Source: CAD feature listing. Evaluate the final solid. Frame: model axes, mm. Give positions to 0.01 mm unless a question says otherwise; leave off trailing zeros. Order: outer loops, then holes, each group sorted by start corner. A loop starts at its lowest first (then second) coordinate and runs counter-clockwise, first axis right, second up.
1) Section C-C, the plane y = 5. Return loops of the section in (x, z).
2) First-contact query: P1, Ø1, axis at x = 1.5, y = -6, coming from the -Z side; P2, Ø1, axis at x = 3, z = 2.5, coming from the -Y side. Flat tips, straight axial feed; report the tip coordinate or a pass-through.
3) Section D-D, the plane z = 2.75. Return loops of the section in (x, y).
4) Section A-A, the plane z = 1.3. Return loops of the section in (x, y), plus the area to 3 significant figures.
5) Material intervals for line 1 (Y direction, x = -1.75, z = 0.9); line 2 (X direction, y = 5.5, z = 1.5); line 3 (Y direction, x = -4.5, z = 1.75), sorted ascending.
6) Section B-B, the plane x = -5.25. Return loops of the section in (y, z), plus the area to 3 significant figures.
```python
from build123d import *

# Parameters (mm, degrees)
SKETCH003_R      = 7.5
PAD003_DEPTH     = 3
CHAMFER_SIZE     = 0.5
EXTRUDE001_DEPTH = 3


with BuildPart() as chamfer_body:
    # Sketch003 → Pad003 (new body)
    with BuildSketch(Plane.XY):
        Circle(SKETCH003_R)
    extrude(amount=PAD003_DEPTH)

    # Chamfer
    chamfer_edges = [chamfer_body.edges().sort_by_distance(p)[0] for p in [
        (-7.5, 0, 3),
    ]]
    chamfer(chamfer_edges, length=CHAMFER_SIZE)


with BuildPart() as common:
    # Sketch005 (on Face3 of Pad003) → Extrude001 (new body)
    with BuildSketch(Plane.XY.offset(3)):
        Polygon((6.55, -3.781644), (6.55, 3.781644), (0, 7.563289), (-6.55, 3.781644), (-6.55, -3.781644), (0, -7.563289), align=None)
    extrude(amount=-EXTRUDE001_DEPTH)

    # Common: intersect Chamfer body
    add(chamfer_body.part, mode=Mode.INTERSECT)


solid = common.part
```
From the geometry:
1. outline: (-4.44, 0) - (4.44, 0) - (4.44, 3) - (-4.44, 3) - close
2. P1: stops at z = 0
2. P2: stops at y = -6.12
3. outline: (-6.55, -3.11) arc R7.25 ccw to (-5.97, -4.12) - (-0.58, -7.23) arc R7.25 ccw to (0.58, -7.23) - (5.97, -4.12) arc R7.25 ccw to (6.55, -3.11) - (6.55, 3.11) arc R7.25 ccw to (5.97, 4.12) - (0.58, 7.23) arc R7.25 ccw to (-0.58, 7.23) - (-5.97, 4.12) arc R7.25 ccw to (-6.55, 3.11) - close
4. outline: (-6.55, -3.65) arc R7.5 ccw to (-6.44, -3.85) - (-0.11, -7.5) arc R7.5 ccw to (0.11, -7.5) - (6.44, -3.85) arc R7.5 ccw to (6.55, -3.65) - (6.55, 3.65) arc R7.5 ccw to (6.44, 3.85) - (0.11, 7.5) arc R7.5 ccw to (-0.11, 7.5) - (-6.44, 3.85) arc R7.5 ccw to (-6.55, 3.65) - close
4. area: 149 mm2
5. line 1: y = -6.55 to 6.55
5. line 2: x = -3.57 to 3.57
5. line 3: y = -4.97 to 4.97
6. outline: (-4.53, 0) - (4.53, 0) - (4.53, 3) - (-4.53, 3) - close
6. area: 27.2 mm2
